Geometry check sheet. Reference: the model listing, model coordinates, mm. Coordinates: 2 decimals unless noted, no trailing zeros. Order: outer loops, then holes, each group sorted by start corner. A loop starts at its lowest first (then second) coordinate and runs counter-clockwise, first axis right, second up. Notation, with made-up numbers: M 26.5,-36 L 79.5,-36 A26 ccw 79.5,-17 Z; hole C 8.25,11.25 d9. An arc over 180 degrees is marked long. One line per item, written item: value. Start each with the question number.
1) Sectioned sample at D-D, the plane z = 0. State how many separate pieces and enclosed holes the cut face has, then the cut area to 3 significant figures.
2) Sectioned sample at A-A, the plane x = 241. Enter the section's corners in (y, z), then the cut area to 3 significant figures.
3) Thickness scan on L1, parallel to X at y = 9.65, z = 0; L2, parallel to Y at x = 208, z = -0.5; L3, parallel to Z at x = 64, y = -7. Record the ranges inside material, lowest first. Write a range as from..to.
4) Sectioned sample at B-B, the plane y = 6.5. Enter the section's corners in (x, z), then the cut area to 3 significant figures.
5) Go/stop test with flat-tipped pins: P1, Ø5, axis at y = -8, z = -3.5, coming from the -X side; P2, Ø3, axis at x = 141, z = 0, coming from the -Y side. Record where each tip stops, or that it passes through.
6) Sectioned sample at C-C, the plane x = 115.5. Enter the section's corners in (y, z).
```python
from build123d import *

# Parameters (mm, degrees)
SKETCH1_W           = 10
SKETCH1_H           = 20
SKETCH1_W_2         = 8
SKETCH1_H_2         = 18
BOSS_EXTRUDE1_DEPTH = 250
SKETCH2_R           = 2.5
CUT_EXTRUDE1_DEPTH  = 20
SKETCH3_R           = 2.5
CUT_EXTRUDE2_DEPTH  = 20


with BuildPart() as part:
    # Sketch1 → Boss-Extrude1 (new body)
    with BuildSketch(Plane(origin=(0, 0, 0), x_dir=(0, 0, -1), z_dir=(1, 0, 0))):
        Rectangle(SKETCH1_W, SKETCH1_H)
        Rectangle(SKETCH1_W_2, SKETCH1_H_2, mode=Mode.SUBTRACT)
    extrude(amount=BOSS_EXTRUDE1_DEPTH)

    # Sketch2 → Cut-Extrude1 (cut)
    with BuildSketch(Plane(origin=(0, 10, 0), x_dir=(1, 0, 0), z_dir=(0, 1, 0))):
        with Locations(Location((241, 0, 0), (0, 0, 270))):
            Circle(SKETCH2_R)
        with Locations(Location((9, 0, 0), (0, 0, 270))):
            Circle(SKETCH2_R)
    extrude(amount=-CUT_EXTRUDE1_DEPTH, mode=Mode.SUBTRACT)

    # Sketch3 → Cut-Extrude2 (cut)
    with BuildSketch(Plane(origin=(0, 10, 0), x_dir=(1, 0, 0), z_dir=(0, 1, 0))):
        with Locations(Location((109, 0, 0), (0, 0, 270))):
            Circle(SKETCH3_R)
        with Locations(Location((141, 0, 0), (0, 0, 270))):
            Circle(SKETCH3_R)
    extrude(amount=-CUT_EXTRUDE2_DEPTH, mode=Mode.SUBTRACT)


solid = part.part
```
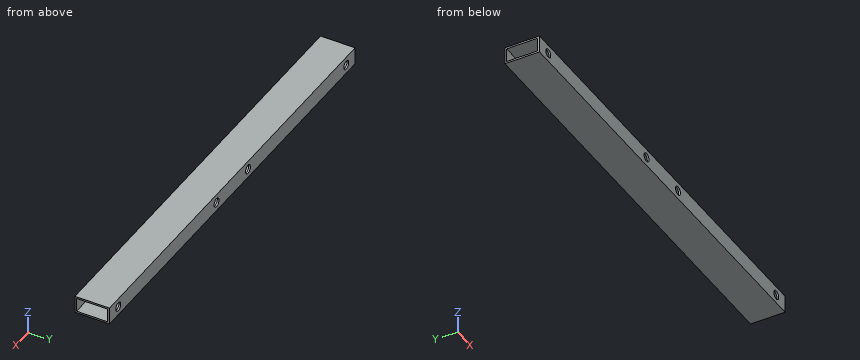
Final values:
1. separate pieces: 10
1. enclosed holes: 0
1. area: 460 mm^2
2. outline: M -10,-5 L 10,-5 L 10,-2.5 L 9,-2.5 L 9,-4 L -9,-4 L -9,-2.5 L -10,-2.5 Z; M -10,2.5 L -9,2.5 L -9,4 L 9,4 L 9,2.5 L 10,2.5 L 10,5 L -10,5 Z
2. area: 46.0 mm^2
3. L1: x = 0..6.5, 11.5..106.5, 111.5..138.5, 143.5..238.5, 243.5..250
3. L2: y = -10..-9, 9..10
3. L3: z = -5..-4, 4..5
4. outline: M 0,-5 L 250,-5 L 250,-4 L 0,-4 Z; M 0,4 L 250,4 L 250,5 L 0,5 Z
4. area: 500 mm^2
5. P1: stops at x = 0
5. P2: passes through
6. outline: M -10,-5 L 10,-5 L 10,5 L -10,5 Z; hole M -9,-4 L 9,-4 L 9,4 L -9,4 Z
